from build123d import *

# Parameters (mm, degrees)
F1_DEPTH = 50
F2_W     = 26.5
F2_H     = 29.9426466227
F2_H_2   = 5
F3_DEPTH = 13
F5_R     = 3
F7_DEPTH = 25
F8_R     = 5


with BuildPart() as f1:
    # F0 (on Front) → F1 (new body)
    with BuildSketch(Plane.XZ):
        Polygon((0, 35), (0, 0.8909322478), (17, 0), (17, 5), (14, 5), (14, 22), (2.5, 22), (2.5, 35), (6.4369898587, 80), (3.9369898587, 80), align=None)
    extrude(amount=F1_DEPTH)

    # F2 (on face) → F3 (cut)
    with BuildSketch(Plane.YZ.offset(17)):
        with Locations((-25, 19.9713233113)):
            Rectangle(F2_W, F2_H)
        with Locations((-25, 2.5)):
            Rectangle(F2_W, F2_H_2)
    extrude(amount=-F3_DEPTH, mode=Mode.SUBTRACT)

    # F5
    f5_edges = [f1.edges().sort_by_distance(p)[0] for p in [
        (0, -25, 0.890932),
        (17, -44.125, 0),
        (17, -5.875, 0),
    ]]
    fillet(f5_edges, radius=F5_R)

    # F6 (on face) → F7 (cut)
    with BuildSketch(Plane(origin=(-0.5578334179, 0, 0.0488041002), x_dir=(0, 1, 0), z_dir=(0.9961946981, 0, -0.0871557427))):
        Polygon((-40, 80.2565964795), (-35, 35.0847037901), (-15, 35.0847037901), (-10, 80.2565964795), align=None)
    extrude(amount=-F7_DEPTH, mode=Mode.SUBTRACT)

    # F8
    f8_edges = [f1.edges().sort_by_distance(p)[0] for p in [
        (5.18699, -50, 80),
        (5.18699, -39.987941, 80),
        (5.18699, -10.012059, 80),
        (5.18699, 0, 80),
        (1.259495, -15, 35.10853),
        (1.259495, -35, 35.10853),
    ]]
    fillet(f8_edges, radius=F8_R)


solid = f1.part
Geometry check sheet. Reference: the model listing, model coordinates, mm. A direction names the side the tool comes from. Give positions to 0.01 mm unless a question says otherwise; leave off trailing zeros. Order: outer loops, then holes, each group sorted by start corner. A loop starts at its lowest first (then second) coordinate and runs counter-clockwise, first axis right, second up. Notation, with made-up numbers: M 79.5,30 L 130.5,30 A20 ccw 130.5,46 Z; hole C -34,24 d11. An arc over 180 degrees is marked long. Use a Markdown table: item, result.
Item 1: Section check C-C (z = 71). Record the cut outline in (x, y), and give its area (3 significant figures).
Answers follow:
| item | result |
|---|---|
| outline | M 3.15,-50 L 5.65,-50 L 5.65,-39 L 3.15,-38.98 Z; M 3.15,-11.02 L 5.65,-11 L 5.65,0 L 3.15,0 Z |
| area | 55.1 mm2 |
Item 2: Depth check by flat-ended pin: P1, Ø3.5, axis at y = -4.5, z = 13, coming from the +X side; P2, Ø0.9, axis at x = 15, y = -44, coming from the +Z side; P3, Ø2, axis at x = 12.5, y = -10, coming from the +Z side. Enter the tip coordinate at first touch or a pass-through.
Answers follow:
| item | result |
|---|---|
| P1 | stops at x = 14 |
| P2 | stops at z = 5 |
| P3 | stops at z = 22 |
Item 3: Material ranges on line 1 along Y through (x, z) = (10.5, 6.5); line 2 along Y through (x, z) = (2, 50.5); line 3 along X through (y, z) = (-19.5, 5), recorded low to high.
Answers follow:
| item | result |
|---|---|
| line 1 | y = -50 to -38.25, -11.75 to 0 |
| line 2 | y = -50 to -36.7, -13.3 to 0 |
| line 3 | x = 0 to 4 |
Item 4: Draft check along Z on faces 1 (the cylindrical face through (5.02, -8.83, 78.76)), 2 (the flat face through (4.44, -44.45, 57.18)), 3 (the cylindrical face through (16.04, -44.21, 0.96)). Enter one of: +Z half, -Z half, draft (parallel to the pull), parting line (faces both ways), or undercut.
Answers follow:
| item | result |
|---|---|
| face 1 | +Z half |
| face 2 | undercut |
| face 3 | -Z half |
Item 5: Section check A-A (z = 14.5). Record the cut outline in (x, y), and give its area (3 significant figures).
Answers follow:
| item | result |
|---|---|
| outline | M 0,-50 L 14,-50 L 14,-38.25 L 4,-38.25 L 4,-11.75 L 14,-11.75 L 14,0 L 0,0 Z |
| area | 435 mm2 |
Item 6: Section check B-B (x = 11.75). Record the cut outline in (y, z), and give its area (3 significant figures).
Answers follow:
| item | result |
|---|---|
| outline | M -50,0.28 L -38.25,0.28 L -38.25,22 L -50,22 Z; M -11.75,0.28 L 0,0.28 L 0,22 L -11.75,22 Z |
| area | 511 mm2 |
Item 7: Tool access check on faces 4 (the flat face through (4.44, -5.27, 57.18)), 5 (the flat face through (9, -38.25, 11)), 6 (the cylindrical face through (1.356, -33.896, 36.414)). Record the directions out of +Z, -Z, +X, -X, +Y, -Y that give a thin tool (end or side, any length) a straight path to the whole face; none if there is none.
Answers follow:
| item | result |
|---|---|
| face 4 | +X, +Y, -Y |
| face 5 | -Z, +X |
| face 6 | +Z, +X |
Item 8: Section check D-D (y = -2.5). Record the cut outline in (x, z), and give its area (3 significant figures).
Answers follow:
| item | result |
|---|---|
| outline | M 0,3.74 A3 ccw 2.84,0.74 L 13.84,0.17 A3 ccw 17,3.16 L 17,5 L 14,5 L 14,22 L 2.5,22 L 2.5,35 L 6.38,79.33 L 3.88,79.33 L 0,35 Z |
| area | 455 mm2 |
